Read the model definition and answer for the solid it produces. Units are mm, in the model's axes. Coordinates: 2 decimals unless noted, no trailing zeros. Write each loop counter-clockwise with the first axis right and the second up, starting at its lowest first coordinate (ties: lowest second). Pieces come first, ordered by that corner, then holes.
(1) The part is cut by section C-C, the plane z = 2.5. Determine the outline of the cut face in (x, y), and give its area (3 significant figures).
(2) Straight lines are drawn through the part: line 1 along Y through (x, z) = (-264, 3); line 2 along Y through (x, z) = (-107.5, 3); line 3 along X through (y, z) = (-1, 2.5). For each, find the intervals that lie inside material, in ascending order.
(3) Given pin 1 (3 mm diameter, centred on x = -141.5, z = 8, fed in from -Y); pin 2 (17 mm diameter, centred on x = -264, y = 0, fed in from +Z); pin 3 (4 mm diameter, centred on y = 12, z = 10, fed in from -X); pin 4 (1.5 mm diameter, centred on x = -172.5, z = 8, fed in from +Y), each flat-ended and moving along its own axis, determine where each tip first touches the part or whether it passes through.
(4) The part is cut by section D-D, the plane x = -138.5. Determine the outline of the cut face in (y, z), and give its area (3 significant figures).
(5) The part is cut by section B-B, the plane y = 0. Determine the outline of the cut face in (x, z).
(6) The part is cut by section A-A, the plane x = -264. Determine the outline of the cut face in (y, z).
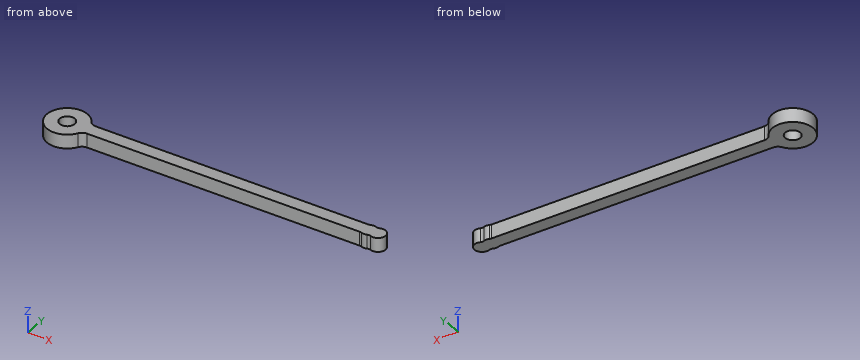
```python
from build123d import *

# Parameters (mm, degrees)
SKETCH_R  = 6.5
PAD_DEPTH = 12


with BuildPart() as part:
    # Sketch → Pad (new body)
    with BuildSketch(Plane.XY):
        with BuildLine():
            ThreePointArc((-1.52381, 6.009865), (-3.999998, 6.5), (-6.476186, 6.009867))
            ThreePointArc((-7.999993, 5.708247), (-7.223307, 5.784376), (-6.476186, 6.009867))
            Line((-7.999993, 5.708247), (-243.337021, 5.708247))
            ThreePointArc((-248.933244, 8.901847), (-246.558697, 6.562824), (-243.337021, 5.708247))
            ThreePointArc((-248.933244, 8.901847), (-281.5, 0), (-248.933244, -8.901847))
            ThreePointArc((-243.337021, -5.708247), (-246.558697, -6.562824), (-248.933244, -8.901847))
            Line((-7.999993, -5.708247), (-243.337021, -5.708247))
            ThreePointArc((-6.476186, -6.009867), (-7.223307, -5.784376), (-7.999993, -5.708247))
            ThreePointArc((-6.476186, -6.009867), (-3.999998, -6.5), (-1.52381, -6.009865))
            ThreePointArc((1.52381, -6.009865), (0, -5.708244), (-1.52381, -6.009865))
            ThreePointArc((1.52381, -6.009865), (10.5, 0), (1.52381, 6.009865))
            ThreePointArc((-1.52381, 6.009865), (0, 5.708244), (1.52381, 6.009865))
        make_face()
        with Locations((-264, 0)):
            Circle(SKETCH_R, mode=Mode.SUBTRACT)
    extrude(amount=PAD_DEPTH)


solid = part.part
```
Computed:
1. outline: (-248.93, -8.9) arc R6.5 cw to (-243.34, -5.71) - (-8, -5.71) arc R4 cw to (-6.48, -6.01) arc R6.5 ccw to (-1.52, -6.01) arc R4 cw to (1.52, -6.01) arc R6.5 ccw (long way) to (1.52, 6.01) arc R4 cw to (-1.52, 6.01) arc R6.5 ccw to (-6.48, 6.01) arc R4 cw to (-8, 5.71) - (-243.34, 5.71) arc R6.5 cw to (-248.93, 8.9) arc R17.5 ccw (long way) to start; hole circle Ø13 at (-264, 0)
1. area: 3,770 mm2
2. line 1: y = -17.5 to -6.5, 6.5 to 17.5
2. line 2: y = -5.71 to 5.71
2. line 3: x = -281.47 to -270.42, -257.58 to 10.42
3. pin 1: stops at y = -5.71
3. pin 2: stops at z = 12
3. pin 3: stops at x = -278.36
3. pin 4: stops at y = 5.71
4. outline: (-5.71, 0) - (5.71, 0) - (5.71, 12) - (-5.71, 12) - close
4. area: 137 mm2
5. outline: (-281.5, 0) - (-270.5, 0) - (-270.5, 12) - (-281.5, 12) - close; (-257.5, 0) - (10.5, 0) - (10.5, 12) - (-257.5, 12) - close
6. outline: (-17.5, 0) - (-6.5, 0) - (-6.5, 12) - (-17.5, 12) - close; (6.5, 0) - (17.5, 0) - (17.5, 12) - (6.5, 12) - close
